Print and shaded views of the part. All mm, measured from the part's lowest x, y and z. A direction names the side the tool comes from. Coordinates: 2 decimals unless noted, no trailing zeros. Order: outer loops, then holes, each group sorted by start corner. A loop starts at its lowest first (then second) coordinate and runs counter-clockwise, first axis right, second up. Notation, with made-up numbers: (27.5, -31) -> (78.5, -31) arc R22 ccw to (78.5, -18) -> close; hole circle Ø6 at (20, 74.5). An arc over 180 degrees is marked (long way). Use one line per item in the form item = value. Start each with the question number.
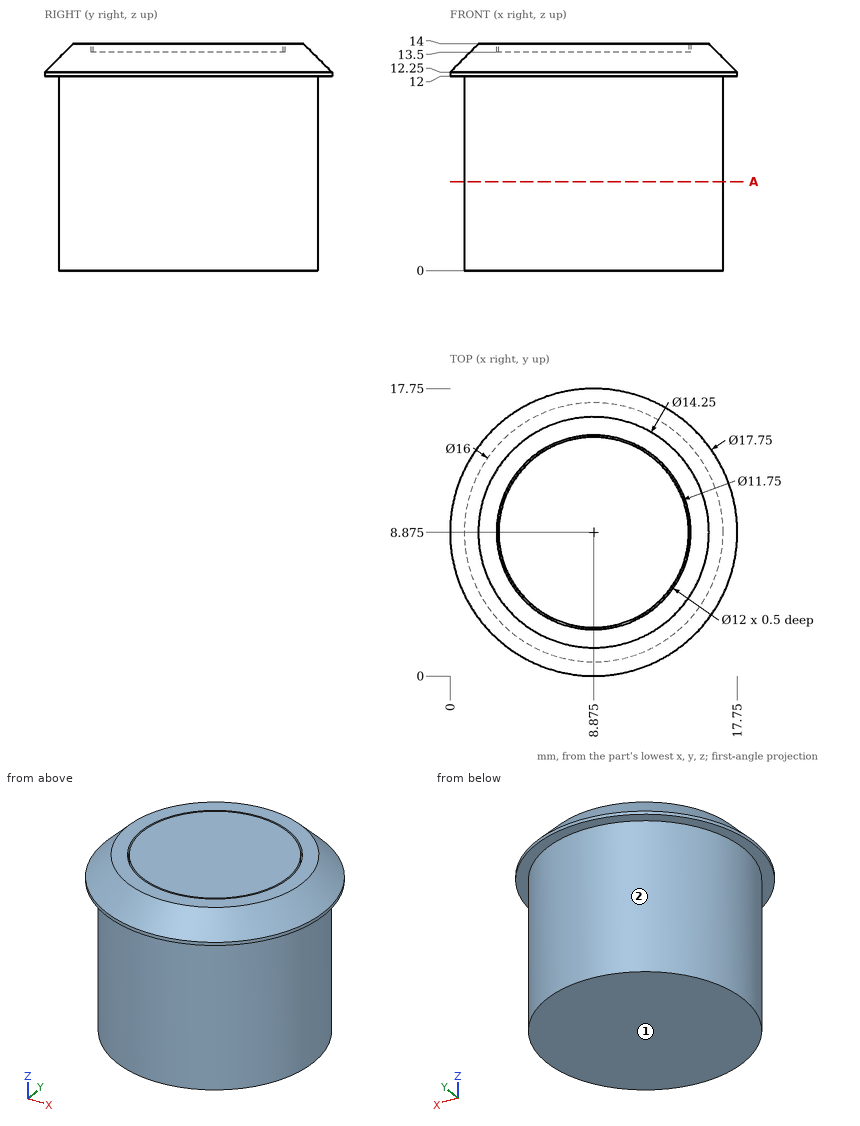
1) Probe L1, parallel to X at y = 12.5, z = 5.5; L2, parallel to X at y = 2, z = 9.75; L3, parallel to Z at x = 16, y = 11.25. List the from-to ranges inside material, lowest first.
2) 3-axis set-ups, long thin cutter, end or side, ignore diameter. For the marked faces 1 and 2: which of +Z, -Z, +X, -X, +Y, -Y reach the whole face in a straight line?
3) Cut at A-A on z = 5.5. Give the cut face in (x, y) (3 decimals), then the cut area to 3 significant figures.
4) Drop flat-ended pins along their axis: P1, Ø1, axis at x = 3, z = 5.5, coming from the -Y side; P2, Ø2, axis at y = 15, z = 7, coming from the +X side; P3, Ø4, axis at x = 13, z = 3.5, coming from the +Y side; P4, Ø9, axis at x = 10.5, y = 7, coming from the -Z side. Give the stop position or say it passes through.
Values follow:
q1.L1 = 1.74 to 16.01
q1.L2 = 4.78 to 12.97
q1.L3 = 0 to 13.61
q2.face_1 = -Z, +X, -X, +Y, -Y
q2.face_2 = -Z
q3.outline = circle Ø16 at (8.875, 8.875)
q3.area = 201 mm^2
q4.P1 = 2.95
q4.P2 = 15.02
q4.P3 = 16.59
q4.P4 = 0
